Build history of the part. All positions in model axes, mm. A direction names the side the tool comes from. Give positions to 0.01 mm unless a question says otherwise; leave off trailing zeros. Order: outer loops, then holes, each group sorted by start corner. A loop starts at its lowest first (then second) coordinate and runs counter-clockwise, first axis right, second up. Notation, with made-up numbers: (79.25, -35) - (86.25, -35) arc R21 cw to (86.25, -31) - close; hole circle Ø10 at (-12, -5). An arc over 180 degrees is marked (long way). Use a Markdown table: item, result. Add a question column.
(1) Which spindle directions (+Z, -Z, +X, -X, +Y, -Y) get a long thin tool onto all of the face, cutting with end or side? Do faces 5 (the face through (57, 88.9, -38)), 6 (the face through (0, 0, -38)), 7 (the face through (-6, 12.7, -38)). Say none if no direction does.
(2) Slice it at B-B (z = -41.5). Write the cut outline in (x, y).
(3) Slice it at A-A (y = 6.35). Write the cut outline in (x, z), then the cut area to 3 significant figures.
(4) Wall check: line 1 (Y direction, x = -69.85, z = -37.25); line 2 (Y direction, x = -22.5, z = -40); line 3 (X direction, y = 83.5, z = -38). Give the ranges that are in metal, low to high.
(5) Flat gauge pins, fed straight in: pin 1 (1 mm diameter, centred on x = 47.5, z = -35.5, fed in from -Y); pin 2 (10 mm diameter, centred on x = -69.85, y = 6.35, fed in from +Z); pin 3 (1 mm diameter, centred on x = 32, z = -33.5, fed in from +Y); pin 4 (6 mm diameter, centred on y = 43, z = -42.5, fed in from -X). Where does each tip first touch, or does it go through?
(6) Slice it at C-C (x = -69.85). Write the cut outline in (y, z).
(7) Slice it at D-D (y = 68). Write the cut outline in (x, z).
(8) Mould opens along X. For faces 1 (the face through (-63.793, 8.257, -38.011)), 2 (the face through (-80.004, 5.999, -38.189)), 3 (the face through (13, 12, -44.45)), 4 (the face through (63.5, 44, -38)) say: +X half, -X half, draft (parallel to the pull), parting line (faces both ways), or undercut.
from build123d import *

# Parameters (mm, degrees)
SKETCH1_W                  = 127
SKETCH1_H                  = 12.7
BOSS_EXTRUDE1_DEPTH        = 12.7
SKETCH9_W                  = 12.7
SKETCH9_H                  = 12.7
BOSS_EXTRUDE2_DEPTH        = 76.2
SKETCH10_R                 = 10.16
BOSS_EXTRUDE3_DEPTH        = 12.7
F_1_2_0_5_DIAMETER_HOLE1_D = 12.7


with BuildPart() as part:
    # Sketch1 → Boss-Extrude1 (new body)
    with BuildSketch(Plane(origin=(0, 0, 0), x_dir=(1, 0, 0), z_dir=(0, 1, 0))):
        with Locations((0, 38.1)):
            Rectangle(SKETCH1_W, SKETCH1_H)
    extrude(amount=BOSS_EXTRUDE1_DEPTH)

    # Sketch9 → Boss-Extrude2 (add)
    with BuildSketch(Plane(origin=(0, 12.7, 0), x_dir=(1, 0, 0), z_dir=(0, 1, 0))):
        with Locations((57.15, 38.1)):
            Rectangle(SKETCH9_W, SKETCH9_H)
    extrude(amount=BOSS_EXTRUDE2_DEPTH)

    # Sketch10 → Boss-Extrude3 (add)
    with BuildSketch(Plane(origin=(0, 0, -44.45), x_dir=(-1, 0, 0), z_dir=(0, 0, -1))):
        with Locations((69.85, 6.35)):
            Circle(SKETCH10_R)
    extrude(amount=-BOSS_EXTRUDE3_DEPTH)

    # 1/2 (0.5) Diameter Hole1 (through all)
    with Locations(Plane(origin=(-69.85, 6.35, -44.45), x_dir=(-1, 0, 0), z_dir=(0, 0, -1))):
        with Locations((0, 0)):
            Hole(F_1_2_0_5_DIAMETER_HOLE1_D / 2)


solid = part.part
Solution:
| question | item | result |
|---|---|---|
| 1 | face 5 | +Z, -Z, +X, -X, +Y |
| 1 | face 6 | +Z, -Z, +X, -Y |
| 1 | face 7 | +Z, -Z, +Y |
| 2 | outline | (-61.92, 0) - (63.5, 0) - (63.5, 88.9) - (50.8, 88.9) - (50.8, 12.7) - (-61.92, 12.7) arc R10.16 ccw (long way) to start; hole circle Ø12.7 at (-69.85, 6.35) |
| 3 | outline | (-80.01, -44.45) - (-76.2, -44.45) - (-76.2, -31.75) - (-80.01, -31.75) - close; (-63.5, -44.45) - (63.5, -44.45) - (63.5, -31.75) - (-63.5, -31.75) - close |
| 3 | area | 1,660 mm2 |
| 4 | line 1 | -3.81 to 0, 12.7 to 16.51 |
| 4 | line 2 | 0 to 12.7 |
| 4 | line 3 | 50.8 to 63.5 |
| 5 | pin 1 | y = 0 |
| 5 | pin 2 | through |
| 5 | pin 3 | y = 12.7 |
| 5 | pin 4 | x = 50.8 |
| 6 | outline | (-3.81, -44.45) - (0, -44.45) - (0, -31.75) - (-3.81, -31.75) - close; (12.7, -44.45) - (16.51, -44.45) - (16.51, -31.75) - (12.7, -31.75) - close |
| 7 | outline | (50.8, -44.45) - (63.5, -44.45) - (63.5, -31.75) - (50.8, -31.75) - close |
| 8 | face 1 | undercut |
| 8 | face 2 | undercut |
| 8 | face 3 | draft |
| 8 | face 4 | +X half |
